```python
from build123d import *

# Parameters (mm, degrees)
SKETCH_1_W          = 40
SKETCH_1_H          = 20
EXTRUDE_1_DEPTH     = 6
SKETCH_2_R          = 2.5
CUT_EXTRUDE_1_DEPTH = 24.151673806
EXTRUDE_START       = -15
EXTRUDE_2_OUTLINE_R = 11
EXTRUDE_2_DEPTH     = 15
EXTRUDE_START_2     = -8
SKETCH_5_R          = 11
SKETCH_5_R_2        = 10
EXTRUDE_3_DEPTH     = 8
EXTRUDE_START_3     = -5
SKETCH_8_W          = 20
SKETCH_8_H          = 28
EXTRUDE_4_DEPTH     = 5
FILLET_1_R          = 1
FILLET_2_R          = 1
SKETCH_9_R          = 2.5
CUT_EXTRUDE_2_DEPTH = 5


# Read off the part's stored shape, not the designer's step: the extrude step
with BuildPart() as part:
    # Sketch 1 → Extrude 1 (new body)
    with BuildSketch(Plane.XY):
        Rectangle(SKETCH_1_W, SKETCH_1_H)
    extrude(amount=EXTRUDE_1_DEPTH)

    # Sketch 2 → Cut-Extrude 1 (cut, through all)
    with BuildSketch(Plane.XY.offset(6)):
        with Locations((10, 0)):
            Circle(SKETCH_2_R)
        with Locations((-1, 0)):
            Circle(SKETCH_2_R)
        with Locations((-12, 0)):
            Circle(SKETCH_2_R)
    extrude(amount=-CUT_EXTRUDE_1_DEPTH, mode=Mode.SUBTRACT)

    # Extrude 2 outline → Extrude 2 (add)
    with BuildSketch(Plane.XY.offset(6).offset(EXTRUDE_START)):
        with BuildLine():
            Line((20, 10), (20, 13.5))
            Line((20, 13.5), (-26.893967141, 13.5))
            Line((-26.893967141, 13.5), (-26.893967141, 13.384337644))
            ThreePointArc((-26.893967141, 13.384337644), (-45, 0), (-26.893967141, -13.384337644))
            Line((-26.893967141, -13.384337644), (-26.893967141, -13.5))
            Line((-26.893967141, -13.5), (20, -13.5))
            Line((20, -13.5), (20, -10))
            Line((20, -10), (-20, -10))
            Line((-20, -10), (-20, -8.660254038))
            ThreePointArc((-20, -8.660254038), (-17, 0), (-20, 8.660254038))
            Line((-20, 8.660254038), (-20, 10))
            Line((-20, 10), (20, 10))
        make_face()
        with Locations((-31, 0)):
            Circle(EXTRUDE_2_OUTLINE_R, mode=Mode.SUBTRACT)
    extrude(amount=EXTRUDE_2_DEPTH)

    # Sketch 5 → Extrude 3 (add)
    with BuildSketch(Plane.XY.offset(6).offset(EXTRUDE_START_2)):
        with Locations((-31, 0)):
            Circle(SKETCH_5_R)
        with Locations((-31, 0)):
            Circle(SKETCH_5_R_2, mode=Mode.SUBTRACT)
    extrude(amount=EXTRUDE_3_DEPTH)

    # Sketch 8 → Extrude 4 (add)
    with BuildSketch(Plane.XY.offset(6).offset(EXTRUDE_START_3)):
        with Locations((-55, 0)):
            Rectangle(SKETCH_8_W, SKETCH_8_H)
        with BuildLine():
            Line((-45, 5.1e-08), (-45, -14))
            Line((-45, -14), (-33.911999365, -13.693803697))
            ThreePointArc((-33.911999365, -13.693803697), (-41.880440979, -8.809994557), (-45, 5.1e-08))
        make_face()
        with BuildLine():
            Line((-45, 14), (-45, 5.1e-08))
            ThreePointArc((-45, 5.1e-08), (-41.968667344, 8.699904408), (-34.187380521, 13.632336755))
            Line((-34.187380521, 13.632336755), (-45, 14))
        make_face()
    extrude(amount=EXTRUDE_4_DEPTH)

    # Fillet 1
    fillet_1_edges = [part.edges().sort_by_distance(p)[0] for p in [
        (-44.999289152, -0.141078849, 1),
    ]]
    fillet(fillet_1_edges, radius=FILLET_1_R)

    # Fillet 2
    fillet_2_edges = [part.edges().sort_by_distance(p)[0] for p in [
        (-65, -14, 3.5),
        (-65, 14, 3.5),
    ]]
    fillet(fillet_2_edges, radius=FILLET_2_R)

    # Sketch 9 → Cut-Extrude 2 (cut)
    with BuildSketch(Plane.XY.offset(6)):
        with Locations((-55, 0)):
            Circle(SKETCH_9_R)
        with Locations((-55, 10)):
            Circle(SKETCH_9_R)
        with Locations((-55, -10)):
            Circle(SKETCH_9_R)
    extrude(amount=-CUT_EXTRUDE_2_DEPTH, mode=Mode.SUBTRACT)


solid = part.part
```
Geometry check sheet. Reference: the model listing, model coordinates, mm. A direction names the side the tool comes from. Coordinates: 2 decimals unless noted, no trailing zeros. Order: outer loops, then holes, each group sorted by start corner. A loop starts at its lowest first (then second) coordinate and runs counter-clockwise, first axis right, second up. Notation, with made-up numbers: (-21, 60) - (7, 60) arc R22 cw to (7, 66) - close; hole circle Ø11 at (25.25, 59.25). An arc over 180 degrees is marked (long way). Answer as a JSON object with one key per item and string values. Group by question number.
Item 1: Depth check by flat-ended pin: pin 1 Ø2.5 at (x, z) = (3.5, -3.5) entering from +Y; pin 2 Ø3 at (x, y) = (-1, 0) entering from -Z; pin 3 Ø0.7 at (y, z) = (9.5, -5.5) entering from +X; pin 4 Ø2 at (x, z) = (-21.5, -1.5) entering from -Y. Enter the tip coordinate at first touch or a pass-through.
Item 2: Sectioned sample at C-C, the plane x = -55. Record the cut outline in (y, z), and give its area (3 significant figures).
Item 3: Draft check along Y on faces 4 (the face through (-52.69, -10.96, 3.54)), 5 (the face through (-23.1, 6.4, 6)), 6 (the face through (-14.5, 0.1, 3)), 7 (the face through (-55, -14, 3)). Enter one of: +Y half, -Y half, draft (parallel to the pull), parting line (faces both ways), or undercut.
Item 4: Scan lines: probe 1 along X at (y, z) = (-0.25, 2); probe 2 along Y at (x, z) = (-55, 3.8); probe 3 along Y at (x, z) = (-31, -1). Record each from-to range of solid material in increasing order.
Item 5: Sectioned sample at B-B, the plane z = -5.25. Record the cut outline in (x, y).
Item 6: Tool access check on faces 1 (the face through (-20.839, -4.213, -5.549)), 2 (the face through (7.5, 0.1, 3)), 3 (the face through (0, -10, -5)). Record the directions out of +Z, -Z, +X, -X, +Y, -Y that give a thin tool (end or side, any length) a straight path to the whole face; none if there is none.
Item 7: Sectioned sample at A-A, the plane x = -1. Record the cut outline in (y, z).
Item 8: Sectioned sample at D-D, the plane z = 2.5. Record the cut outline in (x, y), and give its area (3 significant figures).
Resolved:
{
 "1": {"pin 1": "y = 13.5", "pin 2": "through", "pin 3": "x = -20", "pin 4": "y = -13.5"},
 "2": {"outline": "(-14, 1) - (-12.5, 1) - (-12.5, 6) - (-14, 6) - close; (-7.5, 1) - (-2.5, 1) - (-2.5, 6) - (-7.5, 6) - close; (2.5, 1) - (7.5, 1) - (7.5, 6) - (2.5, 6) - close; (12.5, 1) - (14, 1) - (14, 6) - (12.5, 6) - close", "area": "65.0 mm^2"},
 "3": {"face 4": "undercut", "face 5": "draft", "face 6": "undercut", "face 7": "-Y half"},
 "4": {"probe 1": "-65 to -57.49, -52.51 to -41, -21 to -14.49, -9.51 to -3.49, 1.49 to 7.51, 12.49 to 20", "probe 2": "-14 to -12.5, -7.5 to -2.5, 2.5 to 7.5, 12.5 to 14", "probe 3": "-14 to -10, 10 to 14"},
 "5": {"outline": "(-26.89, -13.5) - (20, -13.5) - (20, -10) - (-20, -10) - (-20, -8.66) arc R14 ccw to (-20, 8.66) - (-20, 10) - (20, 10) - (20, 13.5) - (-26.89, 13.5) - (-26.89, 13.38) arc R14 ccw (long way) to (-26.89, -13.38) - close; hole circle Ø22 at (-31, 0)"},
 "6": {"face 1": "-Z", "face 2": "+Z, -Z", "face 3": "-Z, +X"},
 "7": {"outline": "(-13.5, -9) - (-10, -9) - (-10, 0) - (-2.5, 0) - (-2.5, 6) - (-13.5, 6) - close; (2.5, 0) - (10, 0) - (10, -9) - (13.5, -9) - (13.5, 6) - (2.5, 6) - close"},
 "8": {"outline": "(-65, -13) arc R1 ccw to (-64, -14) - (-45, -14) - (-33.91, -13.69) arc R14 ccw to (-26.89, -13.38) - (-26.89, -13.5) - (20, -13.5) - (20, 13.5) - (-26.89, 13.5) - (-26.89, 13.38) arc R14 ccw to (-34.19, 13.63) - (-45, 14) - (-64, 14) arc R1 ccw to (-65, 13) - close; hole circle Ø5 at (-55, -10); hole circle Ø5 at (-55, 0); hole circle Ø5 at (-55, 10); hole circle Ø20 at (-31, 0); hole circle Ø5 at (-12, 0); hole circle Ø5 at (-1, 0); hole circle Ø5 at (10, 0)", "area": "1,890 mm^2"}
}
